```python
from build123d import *

# Parameters (mm, degrees)
SKETCH1_W                        = 38.1
SKETCH1_H                        = 43.18
BOSS_EXTRUDE1_DEPTH              = 12.7
F_17_64_0_26563_DIAMETER_HOLE1_D = 6.747002
F_1_4_20_TAPPED_HOLE2_D          = 5.1054
F_1_4_20_TAPPED_HOLE2_DEPTH      = 12.7
F_1_4_20_TAPPED_HOLE2_TIP        = 1.533816902
F_1_4_28_TAPPED_HOLE1_D          = 5.4102


with BuildPart() as part:
    # Sketch1 → Boss-Extrude1 (new body)
    with BuildSketch(Plane.XY):
        with Locations((19.05, 21.59)):
            Rectangle(SKETCH1_W, SKETCH1_H)
    extrude(amount=-BOSS_EXTRUDE1_DEPTH)

    # 17/64 (0.26563) Diameter Hole1 (through all)
    with Locations(Plane(origin=(29.21, 36.83, 0), x_dir=(1, 0, 0), z_dir=(0, 0, 1))):
        with Locations((0, 0), (-20.32, 0)):
            Hole(F_17_64_0_26563_DIAMETER_HOLE1_D / 2)

    # 1/4-20 Tapped Hole2
    with Locations(Plane(origin=(0, 27.94, -6.35), x_dir=(0, 0, -1), z_dir=(-1, 0, 0))):
        with Locations((0, 0)):
            Hole(F_1_4_20_TAPPED_HOLE2_D / 2, depth=F_1_4_20_TAPPED_HOLE2_DEPTH)
            with Locations((0, 0, -(F_1_4_20_TAPPED_HOLE2_DEPTH + F_1_4_20_TAPPED_HOLE2_TIP / 2))):  # 118° drill point
                Cone(0, F_1_4_20_TAPPED_HOLE2_D / 2, F_1_4_20_TAPPED_HOLE2_TIP, mode=Mode.SUBTRACT)

    # 1/4-28 Tapped Hole1 (through all)
    with Locations(Plane(origin=(19.05, 15.24, 0), x_dir=(1, 0, 0), z_dir=(0, 0, 1))):
        with Locations((0, 0)):
            Hole(F_1_4_28_TAPPED_HOLE1_D / 2)


solid = part.part
```
Work out the finished part from the listing and answer in its coordinate system (mm). Give positions to 0.01 mm unless a question says otherwise; leave off trailing zeros. Loops run counter-clockwise (first coordinate to the right, second up) from the corner with the lowest first, then second, coordinate; pieces in that order, holes last. Notation, with made-up numbers: (88, 50) -> (146, 50) arc R25 cw to (146, 85) -> close; hole circle Ø5 at (67, 74.5). An arc over 180 degrees is marked (long way). Write item = value, one per line. Start each with the question number.
(1) Find the intervals of material crossed by probe 1 along Z at (x, y) = (4.5, 27.94); probe 2 along X at (y, z) = (37.5, -7.25); probe 3 along Y at (x, z) = (19.05, -7.25), in increasing order. Write a range as from..to.
(2) Find section A-A on x = 8.89. Give the vertices of the cut face in (y, z), and give its area (3 significant figures).
(3) The mould has two halves that part along Y. Classify faces 1 (the cylindrical face through (6.439, 30.432, -6.903)), 2 (the flat face through (19, 22, -12.7)), 3 (the flat face through (19, 43.18, -6)): +Y half, -Y half, draft (parallel to the pull), parting line (faces both ways), or undercut.
(4) Find section C-C on y = 15.24. Give the vertices of the cut face in (x, z), and give its area (3 significant figures).
(5) Find section B-B on y = 36.83. Give the vertices of the cut face in (x, z), and give its area (3 significant figures).
(6) Find section D-D on z = -10.25. Give the vertices of the cut face in (x, y), and give its area (3 significant figures).
From the geometry:
q1.probe_1 = -12.7..-8.9, -3.8..0
q1.probe_2 = 0..5.58, 12.2..25.9, 32.52..38.1
q1.probe_3 = 0..12.53, 17.95..43.18
q2.outline = (0, -12.7) -> (33.46, -12.7) -> (33.46, 0) -> (0, 0) -> close; (40.2, -12.7) -> (43.18, -12.7) -> (43.18, 0) -> (40.2, 0) -> close; hole circle Ø5.11 at (27.94, -6.35)
q2.area = 442 mm^2
q3.face_1 = undercut
q3.face_2 = draft
q3.face_3 = +Y half
q4.outline = (0, -12.7) -> (16.34, -12.7) -> (16.34, 0) -> (0, 0) -> close; (21.76, -12.7) -> (38.1, -12.7) -> (38.1, 0) -> (21.76, 0) -> close
q4.area = 415 mm^2
q5.outline = (0, -12.7) -> (5.52, -12.7) -> (5.52, 0) -> (0, 0) -> close; (12.26, -12.7) -> (25.84, -12.7) -> (25.84, 0) -> (12.26, 0) -> close; (32.58, -12.7) -> (38.1, -12.7) -> (38.1, 0) -> (32.58, 0) -> close
q5.area = 312 mm^2
q6.outline = (0, 0) -> (38.1, 0) -> (38.1, 43.18) -> (0, 43.18) -> close; hole circle Ø6.75 at (8.89, 36.83); hole circle Ø5.41 at (19.05, 15.24); hole circle Ø6.75 at (29.21, 36.83)
q6.area = 1,550 mm^2
